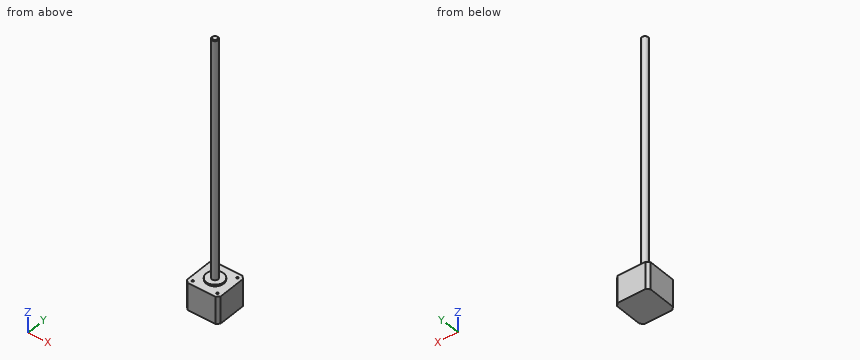
Autodesk Inventor part; units mm, degrees
ref_plane "YZ Plane" through (0, 0, 0) normal (1, 0, 0) x (0, 1, 0)
ref_plane "XZ Plane" through (0, 0, 0) normal (0, 1, 0) x (-1, 0, 0)
ref_plane "XY Plane" through (0, 0, 0) normal (0, 0, 1) x (1, 0, 0)
sketch "Sketch1" plane through (0, 0, 0) normal (0, 0, 1) x (1, 0, 0)
  line L0 (21, -21) -> (-21, -21)
  line L1 (-21, -21) -> (-21, 21)
  line L2 (-21, 21) -> (21, 21)
  line L3 (21, 21) -> (21, -21)
  line L4 (21, -21) -> (-21, 21) construction
  line L5 (-21, -21) -> (21, 21) construction
  point P0 (0, 0)
  dimension "d0" = 42
extrude "Extrusion1" add sketch "Sketch1" along normal blind 34
chamfer "Chamfer1" distance 3.5 angle 45 4 edges at (-21, 21, 17) (21, 21, 17) (21, -21, 17) (-21, -21, 17)
sketch "Sketch2" plane through (0, 0, 34) normal (0, 0, 1) x (1, 0, 0)
  circle A0 centre (0, 0) radius 11
  dimension "d6" = 22
extrude "Extrusion2" add sketch "Sketch2" along normal blind 2
sketch "Sketch3" plane through (0, 0, 36) normal (0, 0, 1) x (1, 0, 0)
  circle A0 centre (0, 0) radius 4
  dimension "d9" = 8
extrude "Extrusion3" add sketch "Sketch3" along normal blind 300
thread "Thread1"
chamfer "Chamfer2" distance 1 angle 45 1 edges at (-4, 0, 336)
sketch "Sketch4" plane through (0, 0, 34) normal (0, 0, 1) x (1, 0, 0)
  line L0 (-17.5, -21) -> (17.5, -21)
  line L1 (17.5, 21) -> (-17.5, 21)
  line L2 (-21, 17.5) -> (-21, -17.5)
  point P0 (0, 0)
  point P1 (-15.5, 15.5)
  point P2 (-15.5, -15.5)
  point P3 (15.5, -15.5)
  point P4 (15.5, 15.5)
  dimension "d17" = 31
  dimension "d18" = 31
  dimension "d19" = 42
  dimension "d21" = 5.5
  dimension "d22" = 5.5
hole "Hole1" at (-15.5, 15.5, 34) at (-15.5, -15.5, 34) at (15.5, -15.5, 34) at (15.5, 15.5, 34) direction (0, 0, -1) diameter 2.459 depth 8.8 tip angle 118
properties part number "Motor_Z" material "Steel, Alloy"
Read the model definition and answer for the solid it produces. Units are mm, in the model's axes. Give positions to 0.01 mm unless a question says otherwise; leave off trailing zeros. Write each loop counter-clockwise with the first axis right and the second up, starting at its lowest first coordinate (ties: lowest second). Pieces come first, ordered by that corner, then holes. Notation, with made-up numbers: (-2.5, 29) -> (45.5, 29) arc R20 ccw to (45.5, 59) -> close; hole circle Ø10 at (-33, 31.5). An arc over 180 degrees is marked (long way). Answer as a JSON object with one key per item and string values. Group by question number.
1) Find section C-C (z = 293). Write down the section's boundary in (x, y).
2) Each of these flat-tipped pins is pushed along its axis until it touches: P1, Ø3, axis at x = -5, z = 94.5, coming from the -Y side; P2, Ø12, axis at y = -6, z = 121.5, coming from the +X side; P3, Ø3, axis at x = 15.5, y = -15.5, coming from the +Z side; P4, Ø1.5, axis at x = -5.5, z = 143, coming from the +Y side. Where does it stop, or does it pass through?
3) Find section A-A (y = 0). Write down the section's boundary in (x, z), and give its area (3 significant figures).
4) Consider L1, parallel to Y at x = -15.5, z = 30.25; L2, parallel to X at y = -15, z = 27. Determine where each line is inside the solid, lowest interval first. Write a range as from..to.
Values follow:
{
 "1": {"outline": "circle Ø8 at (0, 0)"},
 "2": {"P1": "stops at y = -1.94", "P2": "stops at x = 4", "P3": "stops at z = 34", "P4": "passes through"},
 "3": {"outline": "(-21, 0) -> (21, 0) -> (21, 34) -> (11, 34) -> (11, 36) -> (4, 36) -> (4, 335) -> (3, 336) -> (-3, 336) -> (-4, 335) -> (-4, 36) -> (-11, 36) -> (-11, 34) -> (-21, 34) -> close", "area": "3,870 mm2"},
 "4": {"L1": "y = -21..-16.73, -14.27..14.27, 16.73..21", "L2": "x = -21..-16.62, -14.38..14.38, 16.62..21"}
}
